```python
from build123d import *

# Parameters (mm, degrees)
F0_W     = 300
F0_H     = 200
F1_DEPTH = 50
F2_T     = -4


with BuildPart() as f1:
    # F0 (on Top) → F1 (new body, symmetric)
    with BuildSketch(Plane.XY):
        Rectangle(F0_W, F0_H)
    extrude(amount=F1_DEPTH, both=True)

    # F2
    f2_openings = [f1.faces().sort_by_distance(p)[0] for p in [
        (0, 0, 50),
    ]]
    offset(amount=F2_T, openings=f2_openings)


solid = f1.part
```
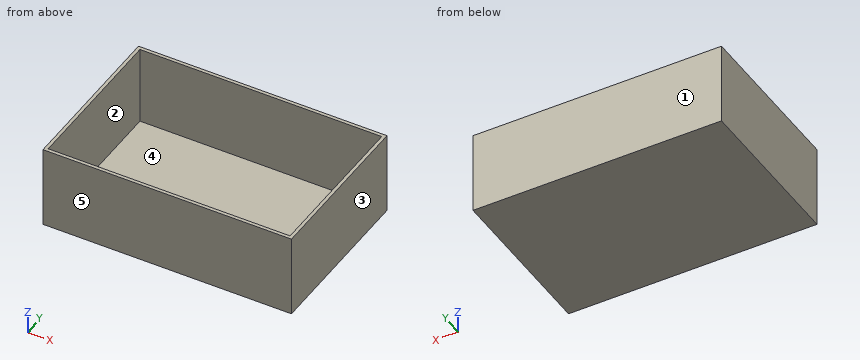
Could you check a few things on this model? Use its own coordinates, in mm. Face numbers are marked on the shaded views. A direction names the side the tool comes from. Round coordinates to 2 decimals unless told otherwise and drop trailing zeros. Loops run counter-clockwise (first coordinate to the right, second up) from the corner with the lowest first, then second, coordinate; pieces in that order, holes last. Notation, with made-up numbers: (67.5, -25) - (118.5, -25) arc R28 ccw to (118.5, 2) - close; hole circle Ø7 at (-15.5, -32.75). An arc over 180 degrees is marked (long way). Answer in a Markdown table with one row per item. Add a question column.
(1) If we section it at B-B (y = -76): Please give me the cut outline in (x, z).
(2) I'm going to push a flat-ended pin straight in: pin 1 (4 mm diameter, centred on x = 92, y = -20.5, fed in from +Z). Where does the tip first touch, or does it pass through?
(3) I need wall thicknesses on line 1 along Y through (x, z) = (-57, 14.5); line 2 along X through (y, z) = (-33, -3); line 3 along Z through (x, y) = (-73.5, 14.5). Which ranges of each line are inside material? Lowest first, please.
(4) If we mould it in two halves opening along Y, with no side actions, what happens to the marked faces 3, 4 and 5? For each: pulls with the +Y half, pulls with the -Y half, needs draft (parallel to the pull), parting line crosses it, or undercut.
(5) For the marked faces 1 and 2, which set-ups out of +Z, -Z, +X, -X, +Y, -Y let a thin tool reach every point of the face, with its end or its side?
(6) If we section it at A-A (z = -32.5): Please give me the cut outline in (x, y), plus the area to 3 significant figures.
(7) If we section it at C-C (x = 34): Please give me the cut outline in (y, z), plus the area to 3 significant figures.
Model answer:
| question | item | result |
|---|---|---|
| 1 | outline | (-150, -50) - (150, -50) - (150, 50) - (146, 50) - (146, -46) - (-146, -46) - (-146, 50) - (-150, 50) - close |
| 2 | pin 1 | stops at z = -46 |
| 3 | line 1 | y = -100 to -96, 96 to 100 |
| 3 | line 2 | x = -150 to -146, 146 to 150 |
| 3 | line 3 | z = -50 to -46 |
| 4 | face 3 | needs draft |
| 4 | face 4 | undercut |
| 4 | face 5 | pulls with the -Y half |
| 5 | face 1 | +Z, -Z, +X, -X, +Y |
| 5 | face 2 | +Z |
| 6 | outline | (-150, -100) - (150, -100) - (150, 100) - (-150, 100) - close; hole (-146, -96) - (146, -96) - (146, 96) - (-146, 96) - close |
| 6 | area | 3,940 mm² |
| 7 | outline | (-100, -50) - (100, -50) - (100, 50) - (96, 50) - (96, -46) - (-96, -46) - (-96, 50) - (-100, 50) - close |
| 7 | area | 1,570 mm² |
